Autodesk Inventor part; units mm, degrees
ref_plane "YZ Plane" through (0, 0, 0) normal (1, 0, 0) x (0, 1, 0)
ref_plane "XZ Plane" through (0, 0, 0) normal (0, 1, 0) x (-1, 0, 0)
ref_plane "XY Plane" through (0, 0, 0) normal (0, 0, 1) x (1, 0, 0)
sketch "Sketch1" plane through (0, 0, 0) normal (0, 1, 0) x (-1, 0, 0)
  point P0 (0, 0)
sketch "Sketch2" plane through (0, 0, 0) normal (0, 1, 0) x (-1, 0, 0)
  line L0 (-51.7536, 0) -> (-51.7536, -6.35)
  line L1 (-51.7536, -6.35) -> (-0.9536, -6.35)
  line L2 (-0.9536, -6.35) -> (-0.9536, 6.35)
  line L3 (-13.6536, 0) -> (-13.6536, 25.4)
  line L4 (-0.9536, 25.4) -> (-0.9536, 6.35)
  line L5 (-13.6536, 0) -> (-51.7536, 0)
  line L6 (-51.7536, 25.4) -> (-51.7536, 31.75)
  line L7 (-51.7536, 31.75) -> (-0.9536, 31.75)
  line L8 (-0.9536, 31.75) -> (-0.9536, 25.4)
  line L9 (-13.6536, 25.4) -> (-51.7536, 25.4)
  point P0 (0, 0)
  dimension "d0" = 50.8
  dimension "d1" = 6.35
  dimension "d2" = 12.7
  dimension "d3" = 25.4
  dimension "d5" = 6.35
revolve "Revolution1" add sketch "Sketch2" angle 360 about axis through (0.9536, 0, 25.4) along (0, 0, -1)
sketch "Sketch3" plane through (0.9536, 0, 31.75) normal (0, 0, 1) x (1, 0, 0)
  circle A0 centre (0, 0) radius 50.8
  point P0 (-0.9536, 0)
hole "Hole1" at (0, 0, 31.75) direction (0, 0, -1) diameter 6.35 end through all
properties part number "spool model"
The listing builds one solid part. Answer for the finished solid, in the listing's coordinates (mm). A direction names the side the tool comes from. Give positions to 0.01 mm unless a question says otherwise; leave off trailing zeros. Loops run counter-clockwise (first coordinate to the right, second up) from the corner with the lowest first, then second, coordinate; pieces in that order, holes last. Notation, with made-up numbers: (26.5, 26) - (40.5, 26) arc R34 ccw to (40.5, 62) - close; hole circle Ø2 at (63, 33). An arc over 180 degrees is marked (long way). Write each question's results on one line, items separated by ' | '.
1. Find section A-A, the plane y = 0. Write down the section's boundary in (x, z) (3 decimals), then the cut area to 3 significant figures.
Resolved:
outline: (-49.846, -6.35) - (-3.175, -6.35) - (-3.175, 31.75) - (-49.846, 31.75) - (-49.846, 25.4) - (-11.746, 25.4) - (-11.746, 0) - (-49.846, 0) - close; (3.175, -6.35) - (51.754, -6.35) - (51.754, 0) - (13.654, 0) - (13.654, 25.4) - (51.754, 25.4) - (51.754, 31.75) - (3.175, 31.75) - close | area: 1,690 mm^2
2. Find section D-D, the plane x = 0. Write down the section's boundary in (y, z) (3 decimals).
Resolved:
outline: (-50.791, -6.35) - (-3.175, -6.35) - (-3.175, 31.75) - (-50.791, 31.75) - (-50.791, 25.4) - (-12.664, 25.4) - (-12.664, 0) - (-50.791, 0) - close; (3.175, -6.35) - (50.791, -6.35) - (50.791, 0) - (12.664, 0) - (12.664, 25.4) - (50.791, 25.4) - (50.791, 31.75) - (3.175, 31.75) - close
3. Find section C-C, the plane z = 5. Write down the section's boundary in (x, y) (3 decimals).
Resolved:
outline: circle Ø25.4 at (0.954, 0); hole circle Ø6.35 at (0, 0)
4. Which of the six approach directions +Z, -Z, +X, -X, +Y, -Y give full straight-line access (tool end or side, diameter ignored) to faces 1 (the face through (0, 11, -6.35)), 2 (the face through (12, 11, 25.4))?
Resolved:
face 1: -Z, +X, -X, +Y, -Y | face 2: none
5. For a pull along X with two mould halves and no side action, classify faces 3 (the face through (6.81, -11.27, 12.88)), 4 (the face through (12, 11, 0)), 5 (the face through (3.1, 0.69, 12.43)) as +X half, -X half, draft (parallel to the pull), parting line (faces both ways), or undercut.
Resolved:
face 3: parting line | face 4: draft | face 5: undercut
6. Flat-ended cylindrical pins translate along their axes: P1, Ø6, axis at y = 7.5, z = 14.5, coming from the +X side; P2, Ø6, axis at y = 32.5, z = 0, coming from the -X side; P3, Ø8, axis at y = 8, z = 1, coming from the +X side. Find the tip coordinate at first contact, or state that the pin passes through.
Resolved:
P1: stops at x = 12.83 | P2: stops at x = -40.4 | P3: stops at x = 51.59
7. Consider probe 1 along Z at (x, y) = (-45, -12); probe 2 along X at (y, z) = (0, 6) (3 decimals); probe 3 along Y at (x, z) = (0, 15) (3 decimals). Determine where each line is inside the solid, lowest interval first. Write a range as from..to.
Resolved:
probe 1: z = -6.35..0, 25.4..31.75 | probe 2: x = -11.746..-3.175, 3.175..13.654 | probe 3: y = -12.664..-3.175, 3.175..12.664
8. Find section B-B, the plane x = -31.5. Write down the section's boundary in (y, z), then the cut area to 3 significant figures.
Resolved:
outline: (-39.08, -6.35) - (39.08, -6.35) - (39.08, 0) - (-39.08, 0) - close; (-39.08, 25.4) - (39.08, 25.4) - (39.08, 31.75) - (-39.08, 31.75) - close | area: 993 mm^2
